Verification items for the finished model (mm, model axes). Give positions to 0.01 mm unless a question says otherwise; leave off trailing zeros. Order: outer loops, then holes, each group sorted by start corner. A loop starts at its lowest first (then second) coordinate and runs counter-clockwise, first axis right, second up.
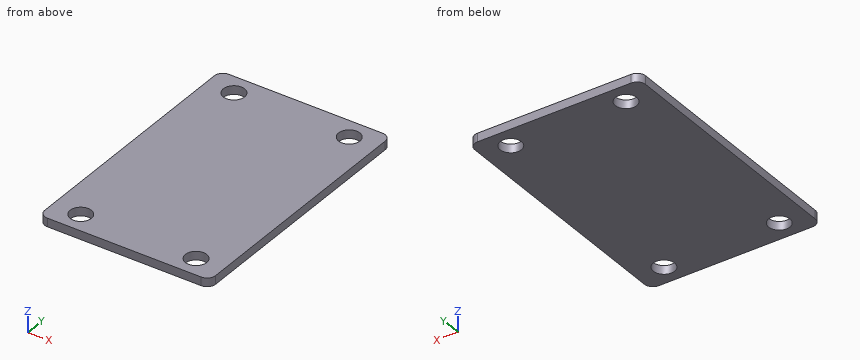
from build123d import *

# Parameters (mm, degrees)
SKETCH1_R           = 1.25
BOSS_EXTRUDE1_DEPTH = 1


with BuildPart() as part:
    # Sketch1 → Boss-Extrude1 (new body)
    with BuildSketch(Plane.XY):
        with BuildLine():
            Line((0, 14.283660896), (0, -7.246695314))
            Line((0, -7.246695314), (0, -14.283660896))
            ThreePointArc((0, -14.283660896), (-0.292893219, -14.990767678), (-1, -15.283660896))
            Line((-1, -15.283660896), (-19, -15.283660896))
            ThreePointArc((-19, -15.283660896), (-19.707106781, -14.990767678), (-20, -14.283660896))
            Line((-20, -14.283660896), (-20, -7.246695314))
            Line((-20, -7.246695314), (-20, 14.283660896))
            ThreePointArc((-20, 14.283660896), (-19.707106781, 14.990767678), (-19, 15.283660896))
            Line((-19, 15.283660896), (-1, 15.283660896))
            ThreePointArc((-1, 15.283660896), (-0.292893219, 14.990767678), (0, 14.283660896))
        make_face()
        with Locations((-16.75, -12.908028273)):
            Circle(SKETCH1_R, mode=Mode.SUBTRACT)
        with Locations((-3.25, -12.908028273)):
            Circle(SKETCH1_R, mode=Mode.SUBTRACT)
        with Locations((-3.25, 12.908028273)):
            Circle(SKETCH1_R, mode=Mode.SUBTRACT)
        with Locations((-16.75, 12.908028273)):
            Circle(SKETCH1_R, mode=Mode.SUBTRACT)
    extrude(amount=BOSS_EXTRUDE1_DEPTH)


solid = part.part
(1) Section check A-A, the plane x = -3.25. Enter the section's corners in (y, z), then the cut area to 3 significant figures.
Solved:
outline: (-15.28, 0) - (-14.16, 0) - (-14.16, 1) - (-15.28, 1) - close; (-11.66, 0) - (11.66, 0) - (11.66, 1) - (-11.66, 1) - close; (14.16, 0) - (15.28, 0) - (15.28, 1) - (14.16, 1) - close
area: 25.6 mm2
(2) Section check B-B, the plane y = -12. Enter the section's corners in (x, z), then the cut area to 3 significant figures.
Solved:
outline: (-20, 0) - (-17.61, 0) - (-17.61, 1) - (-20, 1) - close; (-15.89, 0) - (-4.11, 0) - (-4.11, 1) - (-15.89, 1) - close; (-2.39, 0) - (0, 0) - (0, 1) - (-2.39, 1) - close
area: 16.6 mm2
(3) Scan lines: line 1 (Y direction, x = -16.75, z = 0.7); line 2 (X direction, y = 13, z = 0.7); line 3 (Y direction, x = -15.75, z = 0.2). Record each from-to range of solid material in increasing order.
Solved:
line 1: y = -15.28 to -14.16, -11.66 to 11.66, 14.16 to 15.28
line 2: x = -20 to -18, -15.5 to -4.5, -2 to 0
line 3: y = -15.28 to -13.66, -12.16 to 12.16, 13.66 to 15.28
(4) Section check C-C, the plane z = 0.7. Enter the section's corners in (x, y), then the cut area to 3 significant figures.
Solved:
outline: (-20, -14.28) arc R1 ccw to (-19, -15.28) - (-1, -15.28) arc R1 ccw to (0, -14.28) - (0, 14.28) arc R1 ccw to (-1, 15.28) - (-19, 15.28) arc R1 ccw to (-20, 14.28) - close; hole circle Ø2.5 at (-16.75, -12.91); hole circle Ø2.5 at (-16.75, 12.91); hole circle Ø2.5 at (-3.25, -12.91); hole circle Ø2.5 at (-3.25, 12.91)
area: 591 mm2
